Design review of the part built by this model. Coordinates are the model's own, in mm. A direction names the side the tool comes from. Coordinates: 2 decimals unless noted, no trailing zeros. Write each loop counter-clockwise with the first axis right and the second up, starting at its lowest first coordinate (ties: lowest second). Pieces come first, ordered by that corner, then holes.
Q1. For faces 1 (the flat face through (-11.427, -1, -45)), 2 (the flat face through (3.15, -13, -7)), 3 (the flat face through (-11, -2.54, -5)), list the 3-axis set-ups (+Z, -Z, +X, -X, +Y, -Y) from which the entire face can be reached by the end or side of a thin tool; tool diameter is ignored.
Q2. Take a section at B-B, the plane x = -17. Write out the cut boundary in (y, z), plus the area to 3 significant figures.
Q3. For pin 1 Ø4 at (x, z) = (-5.32, 39.85) entering from -Y; pin 2 Ø8 at (y, z) = (-15.5, 25) entering from -X, all flat-tipped, find the tip position at first contact; note any pin that passes through.
Q4. Take a section at C-C, the plane y = -17. Write out the cut boundary in (x, z), plus the area to 3 significant figures.
Q5. For L1, parallel to Z at x = -10, y = -1.25; L2, parallel to Y at x = -15.25, z = -42.5; L3, parallel to X at y = -19, z = 3.5, list the stretches that pass through material, from the lowest coordinate up.
Q6. Take a section at A-A, the plane z = 30. Write out the cut boundary in (x, y).
Q7. The part is to be moulded in two halves that separate along X. For faces 4 (the cylindrical face through (-9.98, -1.29, -20.17)), 5 (the flat face through (-22.25, -1, -7)), 6 (the flat face through (-5, -2, -56.665)), say which applies: released by +X, released by -X, zero draft, split by the parting line, or undercut.
from build123d import *

# Parameters (mm, degrees)
F0_W     = 25.4
F0_H     = 101.6
F1_DEPTH = 25.4
F2_T     = -2.54
F4_D     = 3.175
F5_D     = 3.175
F3_W     = 3.302
F3_H     = 3.302
F6_DEPTH = 10.16


with BuildPart() as f1:
    # F0 (on Front) → F1 (new body)
    with BuildSketch(Plane.XZ):
        with Locations((-9.550009, -5.865395)):
            Rectangle(F0_W, F0_H)
    extrude(amount=F1_DEPTH)

    # F2
    f2_openings = [f1.faces().sort_by_distance(p)[0] for p in [
        (-9.550009, -25.4, -5.865395),
        (-9.550009, -12.7, 44.934605),
        (-22.250009, -12.7, -5.865395),
        (-9.550009, -12.7, -56.665395),
    ]]
    offset(amount=F2_T, openings=f2_openings)

    # F4 (through all)
    with Locations(Plane(origin=(0, 0, 0), x_dir=(-1, 0, 0), z_dir=(0, 1, 0))):
        with Locations((9.775658, -21.745628), (9.775658, -33.249211)):
            Hole(F4_D / 2)

    # F5 (through all)
    with Locations(Plane(origin=(0, 0, 0), x_dir=(-1, 0, 0), z_dir=(0, 1, 0))):
        with Locations((5.316675, 39.854605), (13.783342, 39.854605)):
            Hole(F5_D / 2)

    # F3 (on face) → F6 (cut)
    with BuildSketch(Plane(origin=(0, 0, 0), x_dir=(-1, 0, 0), z_dir=(0, 1, 0))):
        with Locations((9.775658, -44.752795)):
            Rectangle(F3_W, F3_H)
    extrude(amount=-F6_DEPTH, mode=Mode.SUBTRACT)


solid = f1.part
Responses:
1. face 1: +Y, -Y
1. face 2: +Z, -Z, +X, +Y, -Y
1. face 3: +Z, -Z, -X, -Y
2. outline: (-2.54, -56.67) - (0, -56.67) - (0, 44.93) - (-2.54, 44.93) - close
2. area: 258 mm2
3. pin 1: stops at y = -2.54
3. pin 2: stops at x = 0.61
4. outline: (0.61, -56.67) - (3.15, -56.67) - (3.15, 44.93) - (0.61, 44.93) - close
4. area: 258 mm2
5. L1: z = -56.67 to -46.4, -43.1 to -34.82, -31.68 to -23.32, -20.17 to 44.93
5. L2: y = -2.54 to 0
5. L3: x = 0.61 to 3.15
6. outline: (-22.25, -2.54) - (0.61, -2.54) - (0.61, -25.4) - (3.15, -25.4) - (3.15, 0) - (-22.25, 0) - close
7. face 4: undercut
7. face 5: released by -X
7. face 6: zero draft
